The model under review builds one solid part; all positions refer to its coordinate system, in mm. Face numbers are marked on the shaded views. A direction names the side the tool comes from. Give positions to 0.01 mm unless a question says otherwise; leave off trailing zeros. Write each loop counter-clockwise with the first axis right and the second up, starting at its lowest first coordinate (ties: lowest second). Pieces come first, ordered by that corner, then holes. Notation, with made-up numbers: M 11,70 L 21,70 A11 ccw 21,87 Z; hole C 45,54.5 d9. An arc over 180 degrees is marked long. Write each question's results on one line, items separated by ' | '. Start each with the question number.
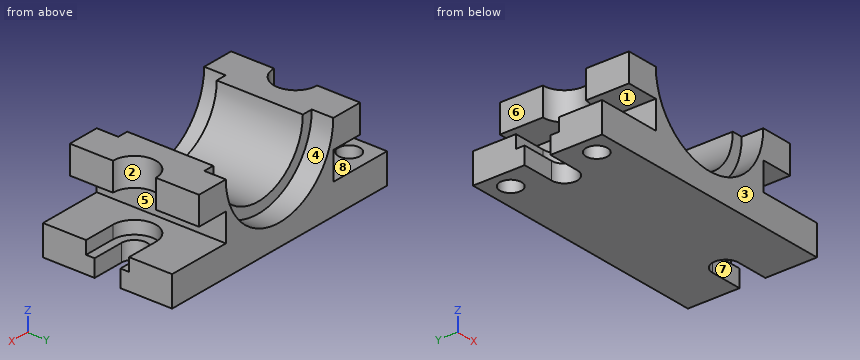
from build123d import *

# Parameters (mm, degrees)
F1_DEPTH      = 30
F1_DEPTH_BACK = 30
F3_DEPTH      = 10
F5_DEPTH      = 10
F7_DEPTH      = 32
F9_DEPTH      = 14
F10_R         = 5
F11_DEPTH     = 15


with BuildPart() as f1:
    # F0 (on Front) → F1 (new body, two sides)
    with BuildSketch(Plane.XZ) as f1_sk:
        with BuildLine():
            Line((45, 7), (45, 20))
            Line((45, 20), (25, 20))
            ThreePointArc((25, 20), (0, -5), (-25, 20))
            Line((-25, 20), (-45, 20))
            Line((-45, 20), (-45, 7))
            Line((-45, 7), (-30, 7))
            Line((-30, 7), (-30, -6))
            Line((-30, -6), (-60, -6))
            Line((-60, -6), (-60, -20))
            Line((-60, -20), (60, -20))
            Line((60, -20), (60, -6))
            Line((60, -6), (30, -6))
            Line((30, -6), (30, 7))
            Line((30, 7), (45, 7))
        make_face()
    extrude(amount=F1_DEPTH)
    extrude(f1_sk.sketch, amount=-F1_DEPTH_BACK)

    # F2 (on face) → F3 (cut)
    with BuildSketch(Plane(origin=(0, 30, 0), x_dir=(-1, 0, 0), z_dir=(0, 1, 0))):
        with BuildLine():
            Line((-25, 20), (-30, 20))
            ThreePointArc((-30, 20), (0, -10), (30, 20))
            Line((30, 20), (25, 20))
            ThreePointArc((25, 20), (0, -5), (-25, 20))
        make_face()
    extrude(amount=-F3_DEPTH, mode=Mode.SUBTRACT)

    # F4 (on face) → F5 (cut)
    with BuildSketch(Plane.XZ.offset(30)):
        with BuildLine():
            Line((30, 20), (-30, 20))
            ThreePointArc((-30, 20), (0, -10), (30, 20))
        make_face()
    extrude(amount=-F5_DEPTH, mode=Mode.SUBTRACT)

    # F6 (on face) → F7 (cut)
    with BuildSketch(Plane.XY.offset(20)):
        with BuildLine():
            Line((-45, 10), (-78.402293, 10))
            Line((-78.402293, 10), (-78.402293, -10))
            Line((-78.402293, -10), (-45, -10))
            ThreePointArc((-45, -10), (-35, 0), (-45, 10))
        make_face()
        with BuildLine():
            ThreePointArc((45, 10), (35, 0), (45, -10))
            Line((45, -10), (78.402293, -10))
            Line((78.402293, -10), (78.402293, 10))
            Line((78.402293, 10), (45, 10))
        make_face()
    extrude(amount=-F7_DEPTH, mode=Mode.SUBTRACT)

    # F8 (on face) → F9 (cut)
    with BuildSketch(Plane.XY.offset(-6)):
        with BuildLine():
            Line((-45, 6), (-64, 6))
            Line((-64, 6), (-64, -6))
            Line((-64, -6), (-45, -6))
            ThreePointArc((-45, -6), (-39, 0), (-45, 6))
        make_face()
        with BuildLine():
            ThreePointArc((45, 6), (39, 0), (45, -6))
            Line((45, -6), (64, -6))
            Line((64, -6), (64, 6))
            Line((64, 6), (45, 6))
        make_face()
    extrude(amount=-F9_DEPTH, mode=Mode.SUBTRACT)

    # F10 (on face) → F11 (cut)
    with BuildSketch(Plane.XY.offset(-6)):
        with Locations((-50.948888, 20)):
            Circle(F10_R)
        with Locations((-50.948888, -20)):
            Circle(F10_R)
    extrude(amount=-F11_DEPTH, mode=Mode.SUBTRACT)


solid = f1.part
(1) Machinability: for the marked faces 4, 5, 6, 7 and 8, which of the approach directions +Z, -Z, +X, -X, +Y, -Y give a long, thin tool a straight path to every point of the face, cutting with its end or side? Answer none if there is none.
(2) Add section C-C (y = -23). State the section outline as (x, z) points.
(3) Draft analysis for pull direction Y (two halves, no side actions). For the marked faces 1, 2 and 3, state which applies: pulls with the +Y half, pulls with the -Y half, needs draft (parallel to the pull), parting line crosses it, or undercut.
(4) Wall thickness on L1, parallel to Z at x = -33.5, y = -7; L2, parallel to X at y = -4, z = 8; L3, parallel to Y at x = -39.5, z = -8.5: over which ranges is each line inside the solid? List them lowest first.
(5) Add section D-D (x = -23). State the section outline as (y, z) points.
(6) Add section B-B (z = 2.5). State the section outline as (x, y) points.
(7) Clearance check with flat-ended pins moving along their axes: P1, Ø4, axis at y = 9.5, z = 0, coming from the +X side; P2, Ø10, axis at y = -1, z = 4, coming from the -X side; P3, Ø6.5, axis at y = 18, z = 13.5, coming from the +X side. State where each tip first meets the part, or that it passes through.
(8) Add section A-A (x = 53). State the section outline as (y, z) points.
Calculated:
1) face 4: +Z, +Y | face 5: +X, +Y, -Y | face 6: +Z, -X, +Y, -Y | face 7: +Z, -Z, +X | face 8: -X, +Y, -Y
2) outline: M -60,-20 L -54.95,-20 L -54.95,-6 L -60,-6 Z; M -46.95,-20 L 60,-20 L 60,-6 L 30,-6 L 30,7 L 45,7 L 45,20 L 30,20 A30 cw -30,20 L -45,20 L -45,7 L -30,7 L -30,-6 L -46.95,-6 Z
3) face 1: needs draft | face 2: undercut | face 3: pulls with the -Y half
4) L1: z = -20 to -6, 7 to 20 | L2: x = -35.83 to -21.93, 21.93 to 35.83 | L3: y = -30 to -8.35, 8.35 to 30
5) outline: M -30,-20 L 30,-20 L 30,0.74 L 20,0.74 L 20,10.2 L -20,10.2 L -20,0.74 L -30,0.74 Z
6) outline: M -30,-30 L -24.37,-30 L -24.37,-20 L -17.85,-20 L -17.85,20 L -24.37,20 L -24.37,30 L -30,30 Z; M 17.85,-20 L 24.37,-20 L 24.37,-30 L 30,-30 L 30,30 L 24.37,30 L 24.37,20 L 17.85,20 Z
7) P1: stops at x = 30 | P2: stops at x = -36.34 | P3: stops at x = 45
8) outline: M -30,-20 L -6,-20 L -6,-12 L -10,-12 L -10,-6 L -30,-6 Z; M 6,-20 L 30,-20 L 30,-6 L 10,-6 L 10,-12 L 6,-12 Z
